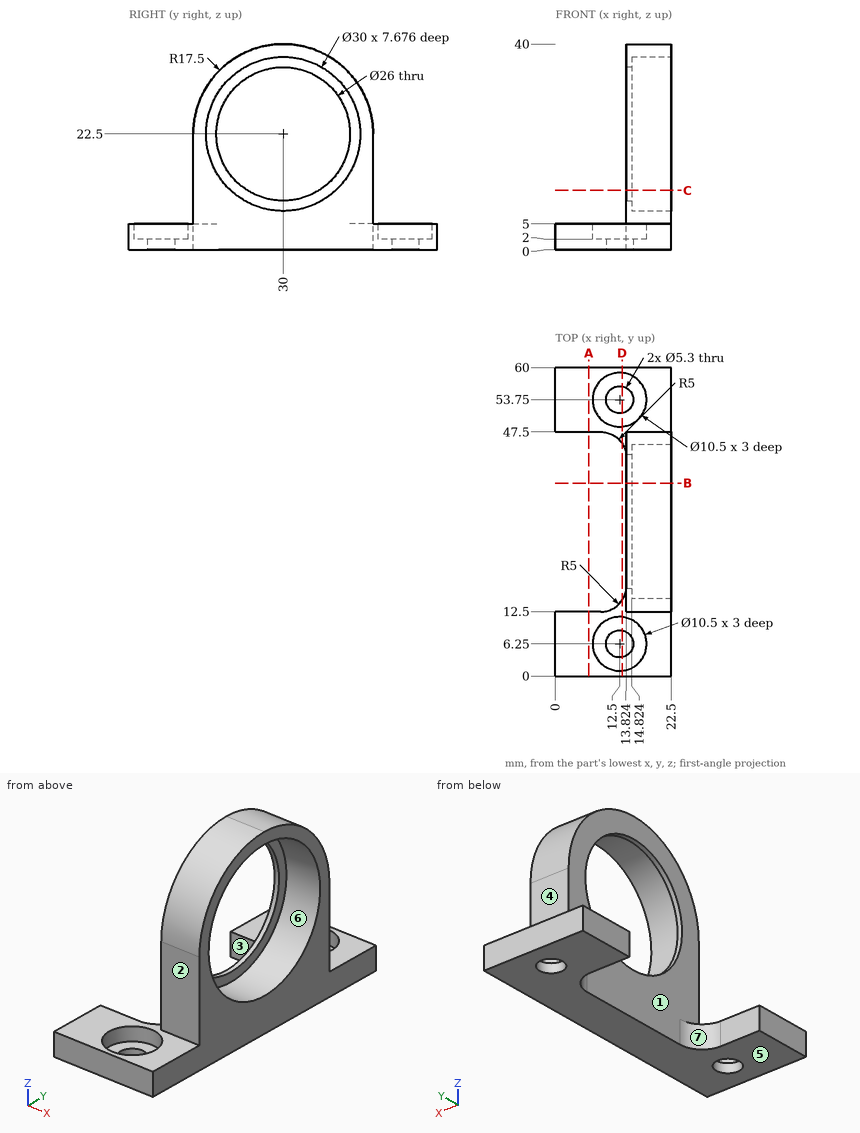
Answer from the drawing. Dimensions are ordinates in mm from the lowest x, y and z of the part. A direction names the side the tool comes from. Round coordinates to 2 decimals unless told otherwise and drop trailing zeros. Loops run counter-clockwise (first coordinate to the right, second up) from the corner with the lowest first, then second, coordinate; pieces in that order, holes last. Notation, with made-up numbers: M 69.5,-32.5 L 122.5,-32.5 A22 cw 122.5,-8.5 Z; hole C 69,-20 d10. An arc over 180 degrees is marked long. One line per question, with ' | ' between items. Start each with the question number.
(1) A cutting plane is placed at B-B on y = 37.5. Write down the section's boundary in (x, z), plus the area to 3 significant figures.
(2) A cutting plane is placed at A-A on x = 6.5. Write down the section's boundary in (y, z).
(3) Find the intervals of material crossed by line 1 (Y direction, x = 12.5, z = 1.4); line 2 (Z direction, x = 14.45, y = 30); line 3 (Y direction, x = 4, z = 4.5), in increasing order.
(4) For a pull along Z with two mould halves and no side action, classify the marked faces 5, 6 and 7 as released by +Z, released by -Z, zero draft, split by the parting line, or undercut.
(5) A tool of negligible diameter and unlimited length cuts with its end or side. For the marked faces 1, 2, 3 and 4, from which of +Z, -Z, +X, -X, +Y, -Y can it reach the whole face along a straight path? Write none if from no direction.
(6) A cutting plane is placed at C-C on z = 11.5. Write down the section's boundary in (x, y).
(7) Flat-ended cylindrical pins translate along their axes: pin 1 Ø1 at (x, z) = (15, 30) entering from -Y; pin 2 Ø8.5 at (x, y) = (12.5, 6.25) entering from +Z; pin 3 Ø8 at (x, y) = (9.5, 8.5) entering from +Z. Find the tip coordinate at first contact, or state that the pin passes through.
(8) A cutting plane is placed at D-D on x = 13. Write down the section's boundary in (y, z).
Geometry check:
1) outline: M 13.82,0 L 22.5,0 L 22.5,9.51 L 14.82,9.51 L 14.82,11.88 L 13.82,11.88 Z; M 13.82,33.12 L 14.82,33.12 L 14.82,35.49 L 22.5,35.49 L 22.5,38.31 L 13.82,38.31 Z | area: 112 mm²
2) outline: M 0,0 L 12.5,0 L 12.5,5 L 0,5 Z; M 47.5,0 L 60,0 L 60,5 L 47.5,5 Z
3) line 1: y = 0 to 3.6, 8.9 to 14.11, 45.89 to 51.1, 56.4 to 60 | line 2: z = 0 to 9.5, 35.5 to 40 | line 3: y = 0 to 12.5, 47.5 to 60
4) face 5: released by -Z | face 6: undercut | face 7: zero draft
5) face 1: +Z, -X | face 2: +Z, +X, -X, -Y | face 3: +Z, -Z, -X | face 4: +Z, +X, -X, +Y
6) outline: M 13.82,12.5 L 22.5,12.5 L 22.5,19.8 L 14.82,19.8 L 14.82,23.07 L 13.82,23.07 Z; M 13.82,36.93 L 14.82,36.93 L 14.82,40.2 L 22.5,40.2 L 22.5,47.5 L 13.82,47.5 Z
7) pin 1: stops at y = 13.96 | pin 2: stops at z = 2 | pin 3: stops at z = 5
8) outline: M 0,0 L 3.65,0 L 3.65,2 L 1.02,2 L 1.02,5 L 0,5 Z; M 8.85,0 L 14.75,0 L 14.75,5 L 11.48,5 L 11.48,2 L 8.85,2 Z; M 45.25,0 L 51.15,0 L 51.15,2 L 48.52,2 L 48.52,5 L 45.25,5 Z; M 56.35,0 L 60,0 L 60,5 L 58.98,5 L 58.98,2 L 56.35,2 Z
